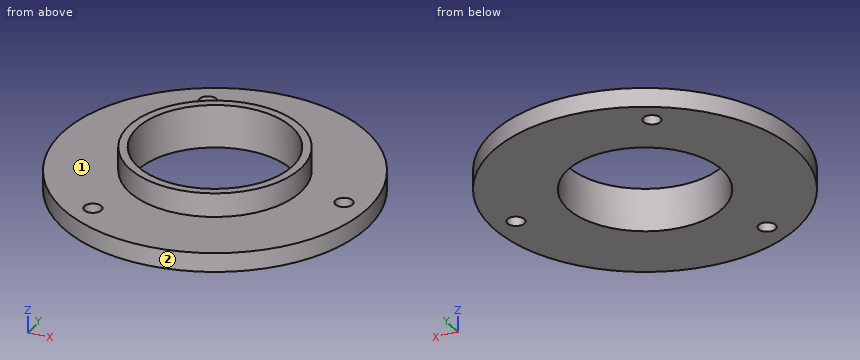
Autodesk Inventor part; units mm, degrees
ref_plane "YZ Plane" through (0, 0, 0) normal (1, 0, 0) x (0, 1, 0)
ref_plane "XZ Plane" through (0, 0, 0) normal (0, 1, 0) x (-1, 0, 0)
ref_plane "XY Plane" through (0, 0, 0) normal (0, 0, 1) x (1, 0, 0)
sketch "Sketch1" plane through (0, 0, 0) normal (0, 0, 1) x (1, 0, 0)
  circle A0 centre (0, 0) radius 16.25
  circle A1 centre (0, 0) radius 18
  circle A2 centre (0, 0) radius 32
  dimension "d0" = 32.5
  dimension "d16" = 64
  dimension "d21" = 36
extrude "Extrusion1" add sketch "Sketch1" along normal blind 4 contours A2
extrude "Extrusion2" add sketch "Sketch1" along normal blind 9 contours A1
sketch "Sketch2" plane through (0, 0, 4) normal (0, 0, 1) x (1, 0, 0)
  circle A0 centre (0, 0) radius 32
  circle A1 centre (27, 0) radius 1.8
  circle A2 centre (-13.5, 23.3827) radius 1.8
  circle A3 centre (-13.5, -23.3827) radius 1.8
  dimension "d8" = 3.6
  dimension "d9" = 27
  dimension "d12" = 360
extrude "Extrusion3" cut sketch "Sketch2" against normal up to surface (4 mm away) contours A1 | A2 | A3
equation "\"d0\" = a"
equation "\"a\" = 32.5"
properties part number "ACO.RODA15-02"
Input: part model. Units: mm. Frame: model coordinates. Face numbers are marked on the shaded views. A direction names the side the tool comes from. Give positions to 0.01 mm unless a question says otherwise; leave off trailing zeros. Order: outer loops, then holes, each group sorted by start corner. A loop starts at its lowest first (then second) coordinate and runs counter-clockwise, first axis right, second up. Notation, with made-up numbers: (-34.75, 10.25) - (5.25, 10.25) arc R18 ccw to (5.25, 25.25) - close; hole circle Ø5 at (85, 71). An arc over 180 degrees is marked (long way). One line per item, written item: value.
1. Pin query (flat end, axial travel): pin 1 Ø4 at (x, y) = (-13.5, 23.38) entering from -Z; pin 2 Ø4 at (x, y) = (-13.5, -23.38) entering from +Z; pin 3 Ø1.5 at (y, z) = (-19.5, 1) entering from -X; pin 4 Ø2 at (x, y) = (27, 0) entering from +Z. Return the tip coordinate at first contact, or that it passes through.
Determined:
pin 1: z = 0
pin 2: z = 4
pin 3: x = -25.93
pin 4: through
2. Cut plane B-B, the plane y = 14. Output: boundary loops of the cut face in (x, z), and give its area (3 significant figures).
Determined:
outline: (-28.77, 0) - (-8.25, 0) - (-8.25, 9) - (-11.31, 9) - (-11.31, 4) - (-28.77, 4) - close; (8.25, 0) - (28.77, 0) - (28.77, 4) - (11.31, 4) - (11.31, 9) - (8.25, 9) - close
area: 195 mm2
3. Line query: probe 1 along Y at (x, z) = (-13.5, 1.35); probe 2 along Z at (x, y) = (-24.5, 14); probe 3 along X at (y, z) = (13.5, 5). Output: solid intervals per line, ascending.
Determined:
probe 1: -29.01 to -25.18, -21.58 to -9.05, 9.05 to 21.58, 25.18 to 29.01
probe 2: 0 to 4
probe 3: -11.91 to -9.05, 9.05 to 11.91
4. Cut plane C-C, the plane z = 6.25. Output: boundary loops of the cut face in (x, y).
Determined:
outline: circle Ø36 at (0, 0); hole circle Ø32.5 at (0, 0)
5. Reachability of the marked faces 1 and 2 from +Z, -Z, +X, -X, +Y, -Y: full face, straight path, thin tool, end or side. Return the list, or none.
Determined:
face 1: +Z
face 2: +Z, -Z
6. Cut plane D-D, the plane x = -13.5. Output: boundary loops of the cut face in (y, z), and give its area (3 significant figures).
Determined:
outline: (-29.01, 0) - (-25.18, 0) - (-25.18, 4) - (-29.01, 4) - close; (-21.58, 0) - (-9.05, 0) - (-9.05, 9) - (-11.91, 9) - (-11.91, 4) - (-21.58, 4) - close; (9.05, 0) - (21.58, 0) - (21.58, 4) - (11.91, 4) - (11.91, 9) - (9.05, 9) - close; (25.18, 0) - (29.01, 0) - (29.01, 4) - (25.18, 4) - close
area: 160 mm2
7. Cut plane A-A, the plane x = 0. Output: boundary loops of the cut face in (y, z).
Determined:
outline: (-32, 0) - (-16.25, 0) - (-16.25, 9) - (-18, 9) - (-18, 4) - (-32, 4) - close; (16.25, 0) - (32, 0) - (32, 4) - (18, 4) - (18, 9) - (16.25, 9) - close
